Geometry check sheet. Reference: the model listing, model coordinates, mm. Face numbers are marked on the shaded views. Give positions to 0.01 mm unless a question says otherwise; leave off trailing zeros. Loops run counter-clockwise (first coordinate to the right, second up) from the corner with the lowest first, then second, coordinate; pieces in that order, holes last. Notation, with made-up numbers: (32.5, -19) -> (76.5, -19) arc R16 ccw to (76.5, -1) -> close; hole circle Ø3 at (50, 55). An arc over 180 degrees is marked (long way). Answer as a JSON object with one key per item and string values.
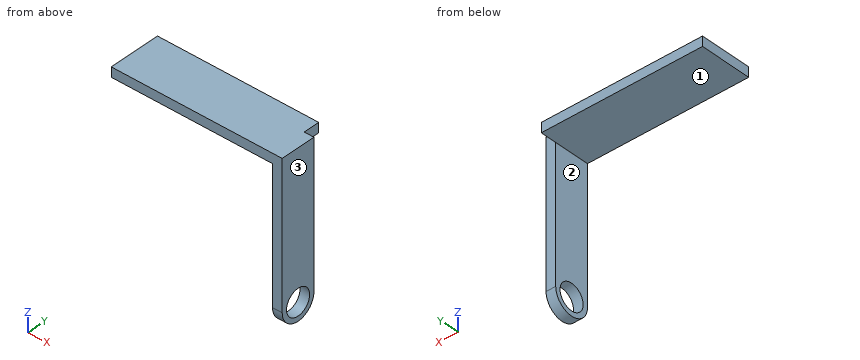
from build123d import *

# Parameters (mm, degrees)
SKETCH069_R     = 0.8
PAD044_DEPTH    = 0.6
SKETCH079_W     = 2.2
SKETCH079_H     = 0.6
PAD040_DEPTH    = 10
PAD040_FACE12_W = 10
PAD040_FACE12_H = 0.6
PAD045_DEPTH    = 1


with BuildPart() as part:
    # Sketch069 → Pad044 (new body)
    with BuildSketch(Plane.YZ):
        with BuildLine():
            Line((0, -8.9), (0, 0))
            Line((0, 0), (2.2, 0))
            Line((2.2, 0), (2.2, -8.9))
            ThreePointArc((0, -8.9), (1.1, -10), (2.2, -8.9))
        make_face()
        with Locations((1.1, -8.9)):
            Circle(SKETCH069_R, mode=Mode.SUBTRACT)
    extrude(amount=PAD044_DEPTH)

    # Sketch079 (on Face6 of Pad044) → Pad040 (join)
    with BuildSketch(Plane(origin=(0, 0, 0), x_dir=(0, 1, 0), z_dir=(-1, 0, 0))):
        with Locations((1.1, 0.3)):
            Rectangle(SKETCH079_W, SKETCH079_H)
    extrude(amount=PAD040_DEPTH)

    # Pad040 Face12 → Pad045 (add)
    with BuildSketch(Plane(origin=(-5, 2.2, -0.3), x_dir=(1, 0, 0), z_dir=(0, 1, 0))):
        Rectangle(PAD040_FACE12_W, PAD040_FACE12_H)
    extrude(amount=PAD045_DEPTH)


with BuildPart() as part_1:
    # Body011 placement: moved
    add(part.part.moved(Location((10, 12.3, 5.5))))


solid = part_1.part
1) Draft check along X on the marked faces 1, 2 and 3. Enter one of: pulls with the +X half, pulls with the -X half, needs draft (parallel to the pull), parting line crosses it, or undercut.
Geometry check:
{"face 1": "needs draft", "face 2": "pulls with the -X half", "face 3": "pulls with the +X half"}
2) Section check C-C on z = 1.5. Record the cut outline in (x, y), plus the area to 3 significant figures.
Geometry check:
{"outline": "(10, 12.3) -> (10.6, 12.3) -> (10.6, 14.5) -> (10, 14.5) -> close", "area": "1.32 mm2"}
3) Section check D-D on y = 14.8. Record the cut outline in (x, z).
Geometry check:
{"outline": "(0, 4.9) -> (10, 4.9) -> (10, 5.5) -> (0, 5.5) -> close"}
4) Material ranges on line 1 along Z through (x, y) = (10.5, 13.4); line 2 along X through (y, z) = (13.7, 4.5); line 3 along Z through (x, y) = (4.25, 13.3), recorded low to high. Write a range as from..to.
Geometry check:
{"line 1": "z = -4.5..-4.2, -2.6..5.5", "line 2": "x = 10..10.6", "line 3": "z = 4.9..5.5"}
5) Section check B-B on z = -3.25. Record the cut outline in (x, y).
Geometry check:
{"outline": "(10, 12.3) -> (10.6, 12.3) -> (10.6, 12.61) -> (10, 12.61) -> close; (10, 14.19) -> (10.6, 14.19) -> (10.6, 14.5) -> (10, 14.5) -> close"}
6) Depth check by flat-ended pin: P1, Ø1.4, axis at y = 13.4, z = -3.4, coming from the -X side; P2, Ø1.8, axis at y = 14, z = 0.5, coming from the -X side; P3, Ø0.7, axis at x = 10, z = 0, coming from the +Y side; P4, Ø1, axis at x = 6, y = 15, coming from the -Z side. Enter the tip coordinate at first touch or a pass-through.
Geometry check:
{"P1": "passes through", "P2": "stops at x = 10", "P3": "stops at y = 14.5", "P4": "stops at z = 4.9"}
7) Section check A-A on y = 13.4. Record the cut outline in (x, z).
Geometry check:
{"outline": "(0, 4.9) -> (10, 4.9) -> (10, -2.6) -> (10.6, -2.6) -> (10.6, 5.5) -> (0, 5.5) -> close; (10, -4.5) -> (10.6, -4.5) -> (10.6, -4.2) -> (10, -4.2) -> close"}
